Geometry: final body of the model. Coordinates: model frame, mm. Face numbers are marked on the shaded views. A direction names the side the tool comes from. Coordinates: 2 decimals unless noted, no trailing zeros. Write each loop counter-clockwise with the first axis right and the second up, starting at its lowest first coordinate (ties: lowest second). Pieces come first, ordered by that corner, then holes.
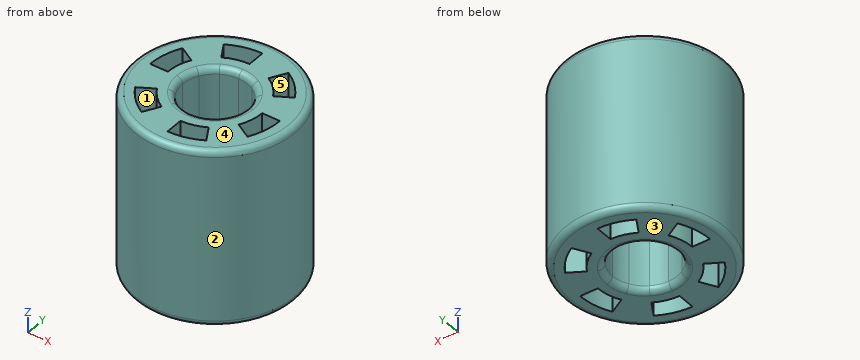
from build123d import *

# Parameters (mm, degrees)
F0_R     = 27
F1_DEPTH = 60
F2_R     = 2


with BuildPart() as f1:
    # F0 (on Top) → F1 (new body)
    with BuildSketch(Plane.XY):
        Circle(F0_R)
        with BuildLine():
            Line((-19.05255878, -10.9999999404), (-13.8564064606, -8))
            ThreePointArc((-13.8564064606, -8), (-11.313708499, -11.313708499), (-8, -13.8564064606))
            Line((-8, -13.8564064606), (-10.9999999404, -19.05255878))
            ThreePointArc((-10.9999999404, -19.05255878), (-15.5563491018, -15.5563491018), (-19.05255878, -10.9999999404))
        make_face(mode=Mode.SUBTRACT)
        with BuildLine():
            Line((0, -21.9999998808), (0, -16))
            ThreePointArc((0, -16), (4.1411047216, -15.4548132206), (8, -13.8564064606))
            Line((8, -13.8564064606), (10.9999999404, -19.05255878))
            ThreePointArc((10.9999999404, -19.05255878), (5.6940189614, -21.2503680632), (0, -21.9999998808))
        make_face(mode=Mode.SUBTRACT)
        with BuildLine():
            Line((16, 0), (21.9999998808, 0))
            ThreePointArc((21.9999998808, 0), (21.2503680632, -5.6940189614), (19.05255878, -10.9999999404))
            Line((19.05255878, -10.9999999404), (13.8564064606, -8))
            ThreePointArc((13.8564064606, -8), (15.4548132206, -4.1411047216), (16, 0))
        make_face(mode=Mode.SUBTRACT)
        with BuildLine():
            Line((-19.05255878, 10.9999999404), (-13.8564064606, 8))
            ThreePointArc((-13.8564064606, 8), (-15.4548132206, 4.1411047216), (-16, 0))
            Line((-16, 0), (-21.9999998808, 0))
            ThreePointArc((-21.9999998808, 0), (-21.2503680632, 5.6940189614), (-19.05255878, 10.9999999404))
        make_face(mode=Mode.SUBTRACT)
        with BuildLine():
            Line((0, 21.9999998808), (0, 16))
            ThreePointArc((0, 16), (-4.1411047216, 15.4548132206), (-8, 13.8564064606))
            Line((-8, 13.8564064606), (-10.9999999404, 19.05255878))
            ThreePointArc((-10.9999999404, 19.05255878), (-5.6940189614, 21.2503680632), (0, 21.9999998808))
        make_face(mode=Mode.SUBTRACT)
        with BuildLine():
            ThreePointArc((9.5262794416, 5.5), (10.6251840892, 2.8470094961), (11, 0))
            ThreePointArc((11, 0), (10.6251840892, -2.8470094961), (9.5262794416, -5.5))
            ThreePointArc((9.5262794416, -5.5), (7.7781745931, -7.7781745931), (5.5, -9.5262794416))
            ThreePointArc((5.5, -9.5262794416), (2.8470094961, -10.6251840892), (0, -11))
            ThreePointArc((0, -11), (-2.8470094961, -10.6251840892), (-5.5, -9.5262794416))
            ThreePointArc((-5.5, -9.5262794416), (-7.7781745931, -7.7781745931), (-9.5262794416, -5.5))
            ThreePointArc((-9.5262794416, -5.5), (-10.6251840892, -2.8470094961), (-11, 0))
            ThreePointArc((-11, 0), (-10.6251840892, 2.8470094961), (-9.5262794416, 5.5))
            ThreePointArc((-9.5262794416, 5.5), (-7.7781745931, 7.7781745931), (-5.5, 9.5262794416))
            ThreePointArc((-5.5, 9.5262794416), (-2.8470094961, 10.6251840892), (0, 11))
            ThreePointArc((0, 11), (2.8470094961, 10.6251840892), (5.5, 9.5262794416))
            ThreePointArc((5.5, 9.5262794416), (7.7781745931, 7.7781745931), (9.5262794416, 5.5))
        make_face(mode=Mode.SUBTRACT)
        with BuildLine():
            Line((19.05255878, 10.9999999404), (13.8564064606, 8))
            ThreePointArc((13.8564064606, 8), (11.313708499, 11.313708499), (8, 13.8564064606))
            Line((8, 13.8564064606), (10.9999999404, 19.05255878))
            ThreePointArc((10.9999999404, 19.05255878), (15.5563491018, 15.5563491018), (19.05255878, 10.9999999404))
        make_face(mode=Mode.SUBTRACT)
    extrude(amount=F1_DEPTH)

    # F2
    f2_edges = [f1.edges().sort_by_distance(p)[0] for p in [
        (-27, 0, 60),
        (-5.5, 9.526279, 60),
        (-27, 0, 0),
        (-5.5, 9.526279, 0),
    ]]
    fillet(f2_edges, radius=F2_R)


solid = f1.part
Item 1: Section B-B, the plane x = -1.5. State how many separate pieces and enclosed holes the cut face has, plus the area to 3 significant figures.
Derived:
separate pieces: 3
enclosed holes: 0
area: 1,560 mm2
Item 2: Pin query (flat end, axial travel): pin 1 (4 mm diameter, centred on x = 17.5, z = 18.5, fed in from +Y); pin 2 (12 mm diameter, centred on x = 4.5, z = 8, fed in from -Y); pin 3 (3 mm diameter, centred on x = -19, z = 39.5, fed in from +Y); pin 4 (5 mm diameter, centred on y = 1, z = 52, fed in from +X). Return the tip coordinate at first contact, or that it passes through.
Derived:
pin 1: stops at y = 22.11
pin 2: stops at y = -27
pin 3: stops at y = 20.56
pin 4: stops at x = 27
Item 3: Pull-direction query (X, two-part tool) for the marked faces 1, 2 and 3; classes: released by +X, released by -X, zero draft, split by the parting line, or undercut.
Derived:
face 1: undercut
face 2: split by the parting line
face 3: zero draft
Item 4: Material intervals for probe 1 along X at (y, z) = (5, 30.5); probe 2 along Y at (x, z) = (18.5, 43.5); probe 3 along Y at (x, z) = (-7, 54), sorted ascending.
Derived:
probe 1: x = -26.53 to -21.42, -15.2 to -9.8, 9.8 to 26.53
probe 2: y = -19.67 to -10.68, 0 to 10.68, 11.91 to 19.67
probe 3: y = -26.08 to -8.49, 8.49 to 14.39, 20.86 to 26.08
Item 5: Section A-A, the plane z = 19.5. Output: boundary loops of the cut face in (x, y).
Derived:
outline: circle Ø54 at (0, 0); hole (-22, 0) - (-16, 0) arc R16 cw to (-13.86, 8) - (-19.05, 11) arc R22 ccw to start; hole (-19.05, -11) arc R22 ccw to (-11, -19.05) - (-8, -13.86) arc R16 cw to (-13.86, -8) - close; hole circle Ø22 at (0, 0); hole (-11, 19.05) - (-8, 13.86) arc R16 cw to (0, 16) - (0, 22) arc R22 ccw to start; hole (0, -22) arc R22 ccw to (11, -19.05) - (8, -13.86) arc R16 cw to (0, -16) - close; hole (8, 13.86) arc R16 cw to (13.86, 8) - (19.05, 11) arc R22 ccw to (11, 19.05) - close; hole (13.86, -8) - (19.05, -11) arc R22 ccw to (22, 0) - (16, 0) arc R16 cw to start
Item 6: Set-up query: the marked faces 4 and 5. Return all of +Z, -Z, +X, -X, +Y, -Y with unobstructed straight access to the full face (end or side cutting, diameter ignored); none if empty.
Derived:
face 4: +Z, +X, -X, +Y, -Y
face 5: +Z, -Z
